Source: three-view drawing plus pictorial views. Frame: mm from the lowest corner of the part. A direction names the side the tool comes from. Give positions to 0.01 mm unless a question says otherwise; leave off trailing zeros. Order: outer loops, then holes, each group sorted by start corner. A loop starts at its lowest first (then second) coordinate and runs counter-clockwise, first axis right, second up.
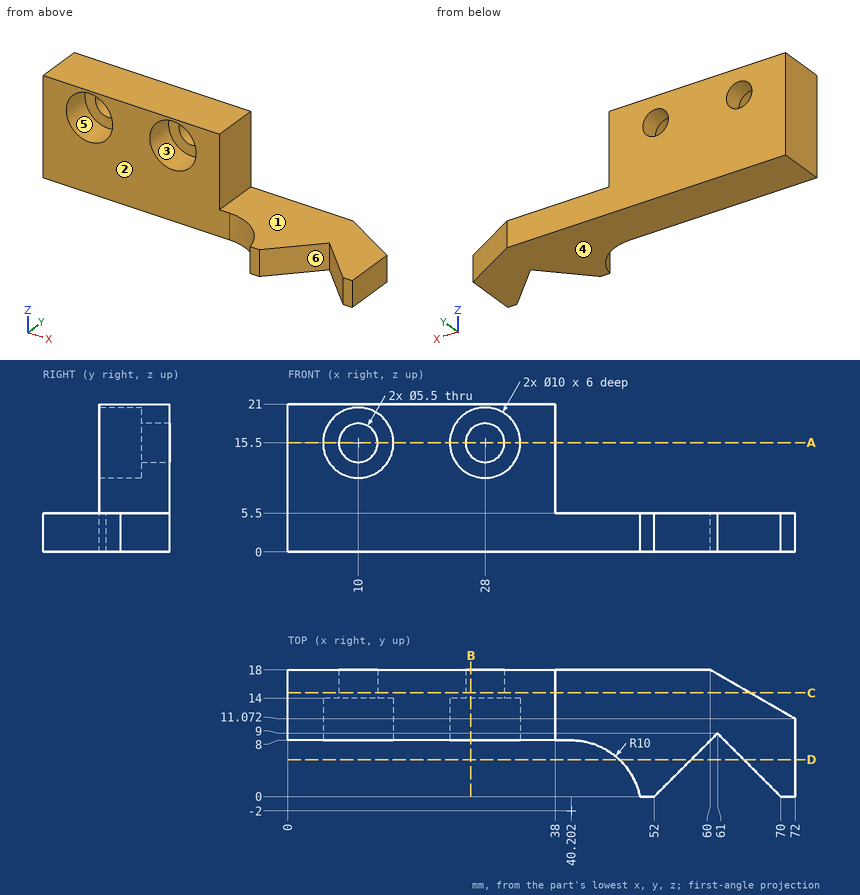
1) Section query A-A on z = 15.5. Output: boundary loops of the cut face in (x, y).
Checks:
outline: (0, 8) - (5, 8) - (5, 14) - (7.25, 14) - (7.25, 18) - (0, 18) - close; (12.75, 14) - (15, 14) - (15, 8) - (23, 8) - (23, 14) - (25.25, 14) - (25.25, 18) - (12.75, 18) - close; (30.75, 14) - (33, 14) - (33, 8) - (38, 8) - (38, 18) - (30.75, 18) - close
2) First-contact query: pin 1 Ø9 at (x, y) = (62, 12.5) entering from +Z; pin 2 Ø11 at (x, z) = (11.5, 16) entering from -Y; pin 3 Ø3 at (y, z) = (13.5, 12.5) entering from +X. Flat tips, straight axial feed; report the tip coordinate or a pass-through.
Checks:
pin 1: stops at z = 5.5
pin 2: stops at y = 8
pin 3: stops at x = 38
3) Section query D-D on y = 5.25. Output: boundary loops of the cut face in (x, z).
Checks:
outline: (47.09, 0) - (57.25, 0) - (57.25, 5.5) - (47.09, 5.5) - close; (64.75, 0) - (72, 0) - (72, 5.5) - (64.75, 5.5) - close
4) Section query C-C on y = 14.75. Output: boundary loops of the cut face in (x, z).
Checks:
outline: (0, 0) - (65.63, 0) - (65.63, 5.5) - (38, 5.5) - (38, 21) - (0, 21) - close; hole circle Ø5.5 at (10, 15.5); hole circle Ø5.5 at (28, 15.5)
5) Pull-direction query (Z, two-part tool) for the marked faces 4, 5 and 6; classes: +Z half, -Z half, draft (parallel to the pull), parting line (faces both ways), or undercut.
Checks:
face 4: -Z half
face 5: undercut
face 6: draft
6) Reachability of the marked faces 1, 2 and 3 from +Z, -Z, +X, -X, +Y, -Y: full face, straight path, thin tool, end or side. Return the list, or none.
Checks:
face 1: +Z, +X, +Y, -Y
face 2: +Z, -Z, -X, -Y
face 3: -Y
7) Ray query, L1, parallel to X at y = 12.15, z = 15.5; L2, parallel to X at y = 14.8, z = 15.5; L3, parallel to Z at x = 61, y = 16. Return the intervals inside material, ascending.
Checks:
L1: x = 0 to 5, 15 to 23, 33 to 38
L2: x = 0 to 7.25, 12.75 to 25.25, 30.75 to 38
L3: z = 0 to 5.5
8) Section query B-B on x = 26. Output: boundary loops of the cut face in (y, z), and give its area (3 significant figures).
Checks:
outline: (8, 0) - (18, 0) - (18, 13.61) - (14, 13.61) - (14, 10.92) - (8, 10.92) - close; (8, 20.08) - (14, 20.08) - (14, 17.39) - (18, 17.39) - (18, 21) - (8, 21) - close
area: 140 mm2
